Design review of the part built by this model. Coordinates are the model's own, in mm. Face numbers are marked on the shaded views. Coordinates: 2 decimals unless noted, no trailing zeros. Order: outer loops, then holes, each group sorted by start corner. A loop starts at its lowest first (then second) coordinate and runs counter-clockwise, first axis right, second up. Notation, with made-up numbers: M 14,50.25 L 25,50.25 A36 ccw 25,86.25 Z; hole C -22,-34.75 d4. An arc over 180 degrees is marked long. Answer as a JSON object with one key per item and string values.
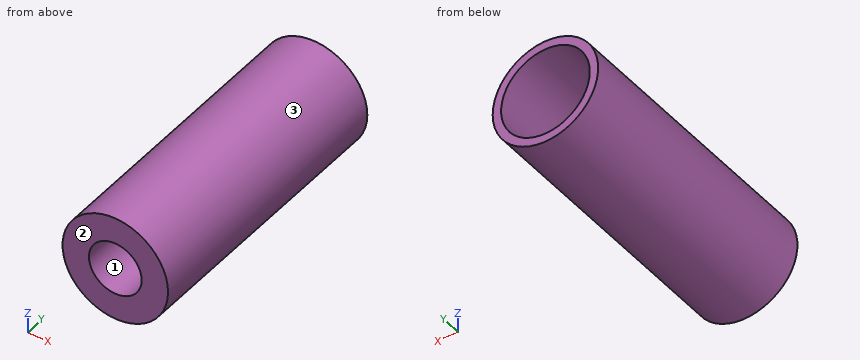
from build123d import *

# Parameters (mm, degrees)
SKETCH1_R                        = 9.525
BOSS_EXTRUDE1_DEPTH              = 50.8
F_16_0_16_DIAMETER_HOLE1_D       = 16
F_16_0_16_DIAMETER_HOLE1_DEPTH   = 25.4
F_16_0_16_DIAMETER_HOLE1_TIP     = 4.806884952
F_3_8_0_375_DIAMETER_HOLE1_D     = 9.525
F_3_8_0_375_DIAMETER_HOLE1_DEPTH = 17.78
F_3_8_0_375_DIAMETER_HOLE1_TIP   = 2.861598698


with BuildPart() as part:
    # Sketch1 → Boss-Extrude1 (new body)
    with BuildSketch(Plane(origin=(0, 0, 0), x_dir=(1, 0, 0), z_dir=(0, 1, 0))):
        Circle(SKETCH1_R)
    extrude(amount=BOSS_EXTRUDE1_DEPTH)

    # Ø16.0 (16) Diameter Hole1
    with Locations(Plane(origin=(0, 50.8, 0), x_dir=(1, 0, 0), z_dir=(0, 1, 0))):
        with Locations((0, 0)):
            Hole(F_16_0_16_DIAMETER_HOLE1_D / 2, depth=F_16_0_16_DIAMETER_HOLE1_DEPTH)
            with Locations((0, 0, -(F_16_0_16_DIAMETER_HOLE1_DEPTH + F_16_0_16_DIAMETER_HOLE1_TIP / 2))):  # 118° drill point
                Cone(0, F_16_0_16_DIAMETER_HOLE1_D / 2, F_16_0_16_DIAMETER_HOLE1_TIP, mode=Mode.SUBTRACT)

    # 3/8 (0.375) Diameter Hole1
    with Locations(Plane(origin=(0, 0, 0), x_dir=(-1, 0, 0), z_dir=(0, -1, 0))):
        with Locations((0, 0)):
            Hole(F_3_8_0_375_DIAMETER_HOLE1_D / 2, depth=F_3_8_0_375_DIAMETER_HOLE1_DEPTH)
            with Locations((0, 0, -(F_3_8_0_375_DIAMETER_HOLE1_DEPTH + F_3_8_0_375_DIAMETER_HOLE1_TIP / 2))):  # 118° drill point
                Cone(0, F_3_8_0_375_DIAMETER_HOLE1_D / 2, F_3_8_0_375_DIAMETER_HOLE1_TIP, mode=Mode.SUBTRACT)


solid = part.part
1) Insertion check: pin 1 Ø5 at (x, y) = (3.5, 27.5) entering from -Z; pin 2 Ø1.5 at (y, z) = (35, 2) entering from -X; pin 3 Ø4 at (y, z) = (6, 7) entering from -X. Each pin has a flat end and moves straight along its axis. Give the tip position at first contact, or say it passes through.
Taken from the geometry:
{"pin 1": "stops at z = -9.47", "pin 2": "stops at x = -9.44", "pin 3": "stops at x = -8.11"}
2) Add section A-A (y = 33.5). State the section outline as (x, z) points (3 decimals), and give its area (3 significant figures).
Taken from the geometry:
{"outline": "C 0,0 d19.05; hole C 0,0 d16", "area": "84.0 mm2"}
3) Mouldability with a two-part tool opening along X and no side actions: class the marked faces 1, 2 and 3 as released by +X, released by -X, zero draft, split by the parting line, or undercut.
Taken from the geometry:
{"face 1": "undercut", "face 2": "zero draft", "face 3": "split by the parting line"}
4) To check wall thickness, follow L1, parallel to Z at x = 0, y = 7 (1 decimal); L2, parallel to X at y = 46.5, z = -6.25; L3, parallel to Z at x = -4, y = 10. State the ranges of each line that lie inside material, in increasing order.
Taken from the geometry:
{"L1": "z = -9.5 to -4.8, 4.8 to 9.5", "L2": "x = -7.19 to -4.99, 4.99 to 7.19", "L3": "z = -8.64 to -2.58, 2.58 to 8.64"}
